Build history of the part. All positions in model axes, mm. A direction names the side the tool comes from. Round coordinates to 2 decimals unless told otherwise and drop trailing zeros. Write each loop counter-clockwise with the first axis right and the second up, starting at its lowest first coordinate (ties: lowest second). Pieces come first, ordered by that corner, then holes. Notation, with made-up numbers: M -13,36 L 40,36 A26 cw 40,50 Z; hole C 51.5,45 d5. An arc over 180 degrees is marked long. Use a Markdown table: item, result.
from build123d import *

# Parameters (mm, degrees)
SKETCH_1_W          = 57
SKETCH_1_H          = 57
EXTRUDE_1_DEPTH     = 76
SKETCH_2_W          = 10
SKETCH_2_H          = 10
CUT_EXTRUDE_1_DEPTH = 70
SKETCH_3_R          = 2.6
CUT_EXTRUDE_2_DEPTH = 90.979320355
FILLET_2_R          = 3
SKETCH_4_R          = 19.05
EXTRUDE_2_DEPTH     = 1.6
SKETCH_5_R          = 4
EXTRUDE_3_DEPTH     = 19.4
CUT_EXTRUDE_START   = -16
CUT_EXTRUDE_3_DEPTH = 16
EXTRUDE_4_DEPTH     = 19.4
FILLET_3_R          = 1
FILLET_4_R          = 1
FILLET_5_R          = 1


with BuildPart() as part:
    # 草图1 → 凸台-拉伸1 (new body)
    with BuildSketch(Plane.XY):
        with Locations((-10.110253485, -0.301500263)):
            Rectangle(SKETCH_1_W, SKETCH_1_H)
    extrude(amount=EXTRUDE_1_DEPTH)

    # 草图2 → 切除-拉伸1 (cut)
    with BuildSketch(Plane(origin=(0, 0, 0), x_dir=(-1, 0, 0), z_dir=(0, 0, -1))):
        with Locations((-13.389746515, 23.198499737)):
            Rectangle(SKETCH_2_W, SKETCH_2_H)
        with Locations((33.610253485, 23.198499737)):
            Rectangle(SKETCH_2_W, SKETCH_2_H)
        with Locations((33.610253485, -23.801500263)):
            Rectangle(SKETCH_2_W, SKETCH_2_H)
        with Locations((-13.389746515, -23.801500263)):
            Rectangle(SKETCH_2_W, SKETCH_2_H)
    extrude(amount=-CUT_EXTRUDE_1_DEPTH, mode=Mode.SUBTRACT)

    # 草图3 → 切除-拉伸2 (cut, through all)
    with BuildSketch(Plane.XY.offset(76)):
        with Locations((13.439746515, 23.248499737)):
            Circle(SKETCH_3_R)
        with Locations((-33.660253485, 23.248499737)):
            Circle(SKETCH_3_R)
        with Locations((-33.660253485, -23.851500263)):
            Circle(SKETCH_3_R)
        with Locations((13.439746515, -23.851500263)):
            Circle(SKETCH_3_R)
    extrude(amount=-CUT_EXTRUDE_2_DEPTH, mode=Mode.SUBTRACT)

    # 圆角2
    fillet_2_edges = [part.edges().sort_by_distance(p)[0] for p in [
        (18.389746515, 18.198499737, 35),
        (8.389746515, 28.198499737, 35),
        (8.389746515, 18.198499737, 35),
        (-38.610253485, 18.198499737, 35),
        (-28.610253485, 18.198499737, 35),
        (-28.610253485, 28.198499737, 35),
        (-38.610253485, -18.801500263, 35),
        (-28.610253485, -28.801500263, 35),
        (-28.610253485, -18.801500263, 35),
        (18.389746515, -18.801500263, 35),
        (8.389746515, -18.801500263, 35),
        (8.389746515, -28.801500263, 35),
        (-38.610253485, 28.198499737, 73),
        (18.389746515, 28.198499737, 73),
        (18.389746515, -28.801500263, 73),
        (-38.610253485, -28.801500263, 73),
    ]]
    fillet(fillet_2_edges, radius=FILLET_2_R)

    # 草图4 → 凸台-拉伸2 (add)
    with BuildSketch(Plane.XY.offset(76)):
        with Locations((-10.110253485, -0.301500263)):
            Circle(SKETCH_4_R)
    extrude(amount=EXTRUDE_2_DEPTH)

    # 草图5 → 凸台-拉伸3 (add)
    with BuildSketch(Plane.XY.offset(77.6)):
        with Locations((-10.110253485, -0.301500263)):
            Circle(SKETCH_5_R)
    extrude(amount=EXTRUDE_3_DEPTH)

    # 草图6 → 切除-拉伸3 (cut)
    with BuildSketch(Plane.XY.offset(97).offset(CUT_EXTRUDE_START)):
        with BuildLine():
            Line((-6.610253485, 1.63499141), (-6.610253485, -2.237991937))
            ThreePointArc((-6.610253485, -2.237991937), (-6.110253485, -0.301500263), (-6.610253485, 1.63499141))
        make_face()
    extrude(amount=CUT_EXTRUDE_3_DEPTH, mode=Mode.SUBTRACT)

    # 草图7 → 凸台-拉伸4 (add)
    with BuildSketch(Plane(origin=(0, 0, 0), x_dir=(-1, 0, 0), z_dir=(0, 0, -1))):
        with BuildLine():
            Line((-12.349002987, -10.964529416), (-18.389746515, -10.964529416))
            Line((-18.389746515, -10.964529416), (-18.389746515, 10.997444042))
            Line((-18.389746515, 10.997444042), (-12.349002987, 10.997444042))
            ThreePointArc((-12.349002987, 10.997444042), (35.110247456, 0.016457313), (-12.349002987, -10.964529416))
        make_face()
    extrude(amount=EXTRUDE_4_DEPTH)

    # 圆角3
    fillet_3_edges = [part.edges().sort_by_distance(p)[0] for p in [
        (18.389746515, 10.997444042, -9.7),
    ]]
    fillet(fillet_3_edges, radius=FILLET_3_R)

    # 圆角4
    fillet_4_edges = [part.edges().sort_by_distance(p)[0] for p in [
        (18.389746515, -10.964529416, -9.7),
    ]]
    fillet(fillet_4_edges, radius=FILLET_4_R)

    # 圆角5
    fillet_5_edges = [part.edges().sort_by_distance(p)[0] for p in [
        (-35.110247456, 0.016457313, -19.4),
    ]]
    fillet(fillet_5_edges, radius=FILLET_5_R)


solid = part.part
Q1. Drill centre lines: L1, parallel to Y at x = -33.5, z = 73; L2, parallel to Z at x = 6, y = 2; L3, parallel to Z at x = -24, y = -21.5. Where is each one in solid material? Low to high.
Response values:
| item | result |
|---|---|
| L1 | y = -28.8 to -26.45, -21.26 to 20.65, 25.84 to 28.2 |
| L2 | z = -19.4 to 77.6 |
| L3 | z = 0 to 76 |
Q2. Cut at B-B on z = 88.5. Give the cut face in (x, y) (1 decimal).
Response values:
| item | result |
|---|---|
| outline | M -6.6,-2.2 L -6.6,1.6 A4 ccw long Z |
Q3. Two-plate mould, pull along X, no slides. Class faces 1 (the cylindrical face through (8.06, 5.42, 76.79)), 2 (the cylindrical face through (-37.75, 27.3, 73.04)), 3 (the cylindrical face through (-31.26, -24.85, 73.04)): +X half, -X half, draft (parallel to the pull), parting line (faces both ways), or undercut.
Response values:
| item | result |
|---|---|
| face 1 | parting line |
| face 2 | -X half |
| face 3 | undercut |
Q4. Drop flat-ended pins along their axis: P1, Ø4, axis at x = 14.5, y = 20.5, coming from the -Z side; P2, Ø1.9, axis at y = 0, z = 90.5, coming from the +X side; P3, Ø1.5, axis at x = 6.5, z = 18, coming from the -Y side. Give the stop position or say it passes through.
Response values:
| item | result |
|---|---|
| P1 | stops at z = 70 |
| P2 | stops at x = -6.61 |
| P3 | stops at y = -28.78 |
Q5. Cut at A-A on z = 54.5. Give the cut face in (x, y), and give its area (3 significant figures).
Response values:
| item | result |
|---|---|
| outline | M -38.61,-15.8 A3 ccw -35.61,-18.8 L -31.61,-18.8 A3 cw -28.61,-21.8 L -28.61,-25.8 A3 ccw -25.61,-28.8 L 5.39,-28.8 A3 ccw 8.39,-25.8 L 8.39,-21.8 A3 cw 11.39,-18.8 L 15.39,-18.8 A3 ccw 18.39,-15.8 L 18.39,15.2 A3 ccw 15.39,18.2 L 11.39,18.2 A3 cw 8.39,21.2 L 8.39,25.2 A3 ccw 5.39,28.2 L -25.61,28.2 A3 ccw -28.61,25.2 L -28.61,21.2 A3 cw -31.61,18.2 L -35.61,18.2 A3 ccw -38.61,15.2 Z |
| area | 2,840 mm2 |
Q6. Which spindle directions (+Z, -Z, +X, -X, +Y, -Y) get a long thin tool onto all of the face, cutting with end or side? Do faces 4 (the flat face through (-30, 0, 76)), 5 (the cylindrical face through (-29.51, -19.66, 35.49)), 6 (the cylindrical face through (7.49, 27.34, 35.49)), 7 (the cylindrical face through (-35.093, 0.957, -9.071)). Say none if no direction does.
Response values:
| item | result |
|---|---|
| face 4 | +Z |
| face 5 | -Z, -X, -Y |
| face 6 | -Z, +X, +Y |
| face 7 | -Z |
